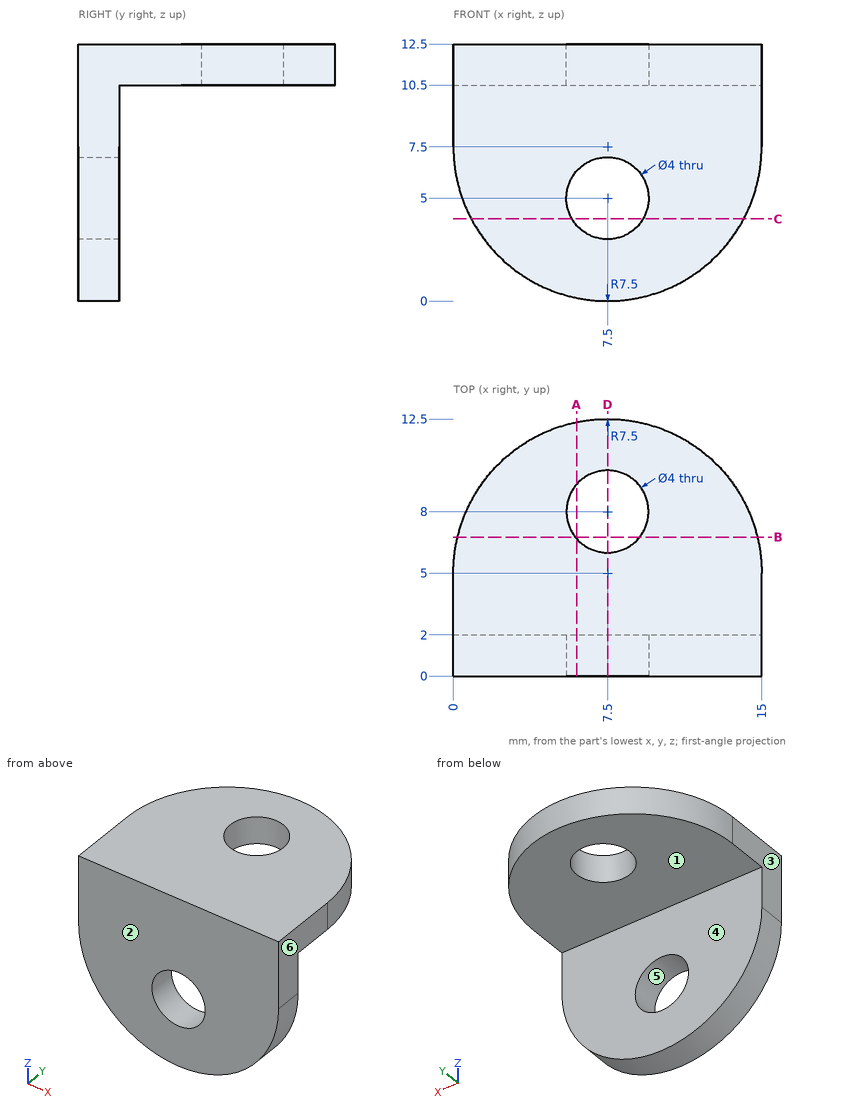
Can you work these out from the drawing? Everything is in mm from the part's minimum corner. A direction names the side the tool comes from. Coordinates: 2 decimals unless noted, no trailing zeros. Order: outer loops, then holes, each group sorted by start corner. A loop starts at its lowest first (then second) coordinate and runs counter-clockwise, first axis right, second up. Notation, with made-up numbers: M 8.5,86.25 L 40.5,86.25 A18 cw 40.5,121.25 Z; hole C 79.5,17.5 d9. An arc over 180 degrees is marked long. Answer as CSV lines item,"result". Start each with the question number.
1. We'd pull the mould along X, two halves only. Please class the marked faces 3, 4, 5 and 6: released by +X, released by -X, zero draft, split by the parting line, or undercut.
2. I need wall thicknesses on line 1 (Y direction, x = 7.5, z = 12.05); line 2 (Y direction, x = 0.5, z = 8.5); line 3 (Z direction, x = 4.5, y = 4.5). Which ranges of each line are inside material? Lowest first, please. Write a range as [from, to].
3. I want a section at A-A, the plane x = 6. Write out the boundary of the cut face in (y, z).
4. For pin 1 (5 mm diameter, centred on x = 6, z = 5, fed in from +Y); pin 2 (5 mm diameter, centred on x = 7.5, y = 8, fed in from -Z); pin 3 (1 mm diameter, centred on x = 8.5, z = 5, fed in from +Y), each with a flat end and sliding along its axis, tell me the tip position at first contact or that it passes through.
5. I want a section at D-D, the plane x = 7.5. Write out the boundary of the cut face in (y, z).
6. I want a section at B-B, the plane y = 6.75. Write out the boundary of the cut face in (x, z), and give its area (3 significant figures).
7. On a 3-axis mill with a long thin cutter (end or side, diameter ignored), from which of +Z, -Z, +X, -X, +Y, -Y can I reach the whole of each face in a straight line? I mean the marked faces 1 and 2. Say none if no direction works.
8. I want a section at C-C, the plane z = 4. Write out the boundary of the cut face in (x, y).
Recorded:
1,face 3,"released by -X"
1,face 4,"zero draft"
1,face 5,"undercut"
1,face 6,"released by +X"
2,line 1,"y = [0, 6], [10, 12.5]"
2,line 2,"y = [0, 2]"
2,line 3,"z = [10.5, 12.5]"
3,outline,"M 0,0.15 L 2,0.15 L 2,3.68 L 0,3.68 Z; M 0,6.32 L 2,6.32 L 2,10.5 L 6.68,10.5 L 6.68,12.5 L 0,12.5 Z; M 9.32,10.5 L 12.35,10.5 L 12.35,12.5 L 9.32,12.5 Z"
4,pin 1,"stops at y = 2"
4,pin 2,"stops at z = 10.5"
4,pin 3,"passes through"
5,outline,"M 0,0 L 2,0 L 2,3 L 0,3 Z; M 0,7 L 2,7 L 2,10.5 L 6,10.5 L 6,12.5 L 0,12.5 Z; M 10,10.5 L 12.5,10.5 L 12.5,12.5 L 10,12.5 Z"
6,outline,"M 0.21,10.5 L 5.94,10.5 L 5.94,12.5 L 0.21,12.5 Z; M 9.06,10.5 L 14.79,10.5 L 14.79,12.5 L 9.06,12.5 Z"
6,area,"22.9 mm2"
7,face 1,"-Z, +X, -X, +Y"
7,face 2,"+Z, -Z, +X, -X, -Y"
8,outline,"M 0.87,0 L 5.77,0 L 5.77,2 L 0.87,2 Z; M 9.23,0 L 14.13,0 L 14.13,2 L 9.23,2 Z"
